The model under review builds one solid part; all positions refer to its coordinate system, in mm. Coordinates: 2 decimals unless noted, no trailing zeros. Loops run counter-clockwise (first coordinate to the right, second up) from the corner with the lowest first, then second, coordinate; pieces in that order, holes last. Notation, with made-up numbers: M 18.25,41.25 L 22.25,41.25 A26 cw 22.25,64.25 Z; hole C 55,63 d11. An arc over 180 degrees is marked long. Write item = value, one per line. Start each with the question number.
Q1. We need section B-B on z = -84. Give the boundary of the cut face in (x, y) (3 decimals), and give its area (3 significant figures).
Q2. Wall thickness on probe 1 along Z at (x, y) = (109.5, -1.4); probe 2 along X at (y, z) = (-1, -96) (3 decimals); probe 3 along X at (y, z) = (-1.05, -6) (1 decimal): over which ranges is each line inside the solid? List them lowest first.
Q3. Clearance check with flat-ended pins moving along their axes: pin 1 Ø3.5 at (x, z) = (5.5, -108.1) entering from -Y; pin 2 Ø2.5 at (x, z) = (135.39, -109.1) entering from -Y. State where each tip first meets the part, or that it passes through.
Q4. We need section A-A on x = 120.5. Give the boundary of the cut face in (y, z).
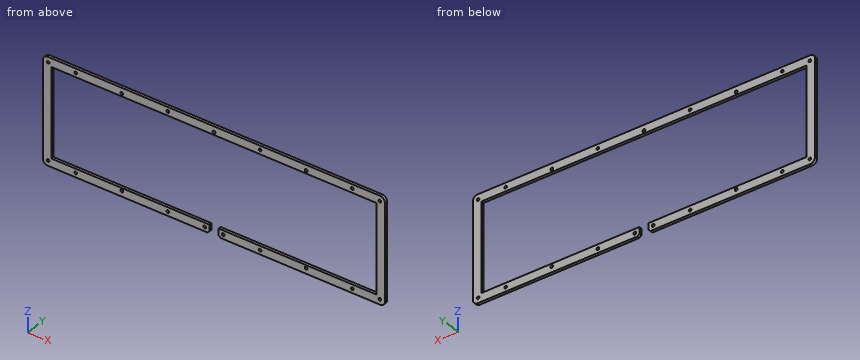
from build123d import *

# Parameters (mm, degrees)
SKETCH1_R           = 1.45
SKETCH1_R_2         = 1.55
BOSS_EXTRUDE1_DEPTH = 3


with BuildPart() as part:
    # Sketch1 → Boss-Extrude1 (new body)
    with BuildSketch(Plane(origin=(0, 0, 0), x_dir=(1, 0, 0), z_dir=(0, 1, 0))):
        with BuildLine():
            Line((6.611e-06, 108.600000663), (6.611e-06, 5.000000663))
            ThreePointArc((6.611e-06, 5.000000663), (1.464472705, 1.464466757), (5.000006611, 6.63e-07))
            Line((5.000006611, 6.63e-07), (365.775006611, 6.63e-07))
            ThreePointArc((365.775006611, 6.63e-07), (369.310540517, 1.464466757), (370.775006611, 5.000000663))
            Line((370.775006611, 5.000000663), (370.775006611, 108.600000663))
            ThreePointArc((370.775006611, 108.600000663), (369.310540517, 112.135534569), (365.775006611, 113.600000663))
            Line((365.775006611, 113.600000663), (192.387506611, 113.600000663))
            Line((192.387506611, 113.600000663), (190.387506611, 111.600000663))
            Line((190.387506611, 111.600000663), (190.387506611, 104.600000663))
            Line((190.387506611, 104.600000663), (361.775006611, 104.600000663))
            Line((361.775006611, 104.600000663), (361.775006611, 9.000000663))
            Line((361.775006611, 9.000000663), (9.000006611, 9.000000663))
            Line((9.000006611, 9.000000663), (9.000006611, 104.600000663))
            Line((9.000006611, 104.600000663), (180.387506611, 104.600000663))
            Line((180.387506611, 104.600000663), (180.387506611, 111.600000663))
            Line((180.387506611, 111.600000663), (178.387506611, 113.600000663))
            Line((178.387506611, 113.600000663), (5.000006611, 113.600000663))
            ThreePointArc((5.000006611, 113.600000663), (1.464472705, 112.135534569), (6.611e-06, 108.600000663))
        make_face()
        with Locations(Location((35.387506611, 4.500000663, 0), (0, 0, 270))):
            Circle(SKETCH1_R, mode=Mode.SUBTRACT)
        with Locations(Location((135.387506611, 4.500000663, 0), (0, 0, 270))):
            Circle(SKETCH1_R, mode=Mode.SUBTRACT)
        with Locations(Location((335.387506611, 4.500000663, 0), (0, 0, 270))):
            Circle(SKETCH1_R, mode=Mode.SUBTRACT)
        with Locations(Location((235.387506611, 4.500000663, 0), (0, 0, 270))):
            Circle(SKETCH1_R, mode=Mode.SUBTRACT)
        with Locations(Location((35.387506611, 109.100000663, 0), (0, 0, 270))):
            Circle(SKETCH1_R, mode=Mode.SUBTRACT)
        with Locations(Location((135.387506611, 109.100000663, 0), (0, 0, 270))):
            Circle(SKETCH1_R, mode=Mode.SUBTRACT)
        with Locations(Location((335.387506611, 109.100000663, 0), (0, 0, 270))):
            Circle(SKETCH1_R, mode=Mode.SUBTRACT)
        with Locations(Location((235.387506611, 109.100000663, 0), (0, 0, 270))):
            Circle(SKETCH1_R, mode=Mode.SUBTRACT)
        with Locations(Location((195.387506611, 109.100000663, 0), (0, 0, 270))):
            Circle(SKETCH1_R_2, mode=Mode.SUBTRACT)
        with Locations(Location((175.387506611, 109.100000663, 0), (0, 0, 270))):
            Circle(SKETCH1_R_2, mode=Mode.SUBTRACT)
        with Locations(Location((5.500006611, 108.100000663, 0), (0, 0, 270))):
            Circle(SKETCH1_R, mode=Mode.SUBTRACT)
        with Locations(Location((5.500006611, 5.500000663, 0), (0, 0, 270))):
            Circle(SKETCH1_R, mode=Mode.SUBTRACT)
        with Locations(Location((365.275006611, 5.500000663, 0), (0, 0, 270))):
            Circle(SKETCH1_R, mode=Mode.SUBTRACT)
        with Locations(Location((365.275006611, 108.100000663, 0), (0, 0, 270))):
            Circle(SKETCH1_R, mode=Mode.SUBTRACT)
        with Locations(Location((85.387506611, 107.600000663, 0), (0, 0, 270))):
            Circle(SKETCH1_R_2, mode=Mode.SUBTRACT)
        with Locations(Location((285.387506611, 107.600000663, 0), (0, 0, 270))):
            Circle(SKETCH1_R_2, mode=Mode.SUBTRACT)
        with Locations(Location((85.387506611, 6.000000663, 0), (0, 0, 270))):
            Circle(SKETCH1_R_2, mode=Mode.SUBTRACT)
        with Locations(Location((185.387506611, 6.000000663, 0), (0, 0, 270))):
            Circle(SKETCH1_R_2, mode=Mode.SUBTRACT)
        with Locations(Location((285.387506611, 6.000000663, 0), (0, 0, 270))):
            Circle(SKETCH1_R_2, mode=Mode.SUBTRACT)
    extrude(amount=-BOSS_EXTRUDE1_DEPTH)


solid = part.part
Returned:
q1.outline = M 0,-3 L 9,-3 L 9,0 L 0,0 Z; M 361.775,-3 L 370.775,-3 L 370.775,0 L 361.775,0 Z
q1.area = 54.0 mm^2
q2.probe_1 = -113.6 to -104.6, -9 to 0
q2.probe_2 = 0 to 9, 361.775 to 370.775
q2.probe_3 = 0 to 4.1, 6.9 to 83.8, 86.9 to 183.8, 186.9 to 283.8, 286.9 to 363.9, 366.6 to 370.8
q3.pin_1 = -3
q3.pin_2 = through
q4.outline = M -3,-113.6 L 0,-113.6 L 0,-104.6 L -3,-104.6 Z; M -3,-9 L 0,-9 L 0,0 L -3,0 Z
